Work out the finished part from the listing and answer in its coordinate system (mm). Face numbers are marked on the shaded views. Round coordinates to 2 decimals unless told otherwise and drop trailing zeros. Loops run counter-clockwise (first coordinate to the right, second up) from the corner with the lowest first, then second, coordinate; pieces in that order, holes last. Notation, with made-up numbers: M 69,19.5 L 75,19.5 A14 cw 75,35.5 Z; hole C -14,-11.5 d8. An arc over 180 degrees is marked long. One line per item, written item: value.
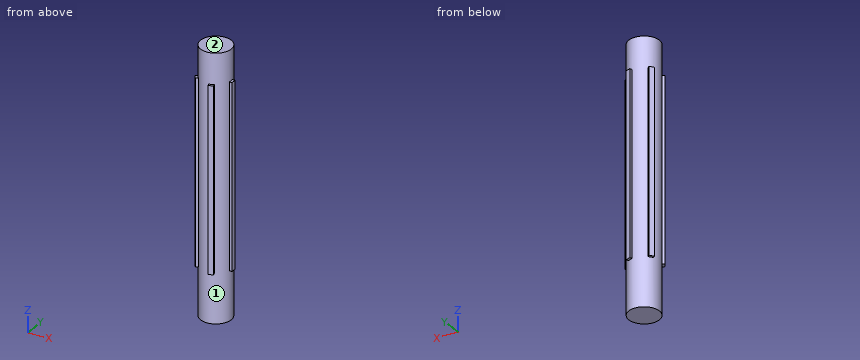
```python
from build123d import *

# Parameters (mm, degrees)
SKETCH1_R           = 12.5
BOSS_EXTRUDE1_DEPTH = 215
BOSS_EXTRUDE2_START = 40
BOSS_EXTRUDE2_DEPTH = 150
CIRPATTERN1_COUNT   = 5


with BuildPart() as part:
    # Sketch1 → Boss-Extrude1 (new body)
    with BuildSketch(Plane.XY):
        Circle(SKETCH1_R)
    extrude(amount=BOSS_EXTRUDE1_DEPTH)

    # Sketch1_3 → Boss-Extrude2 (add)
    with BuildSketch(Plane.XY.offset(BOSS_EXTRUDE2_START)):
        with BuildLine():
            Line((14.5, -2), (14.5, 2))
            Line((14.5, 2), (12.338962679, 2))
            ThreePointArc((12.338962679, 2), (12.459675628, 1.00323639), (12.5, 0))
            ThreePointArc((12.5, 0), (12.459675628, -1.00323639), (12.338962679, -2))
            Line((12.338962679, -2), (14.5, -2))
        make_face()
    boss_extrude2 = extrude(amount=BOSS_EXTRUDE2_DEPTH)

    # CirPattern1: Boss-Extrude2 ×5 about axis
    cirpattern1_axis = Axis((0, 0, 0), (0, 0, 1))
    for i in range(1, CIRPATTERN1_COUNT):
        add(boss_extrude2.rotate(cirpattern1_axis, i * 360 / CIRPATTERN1_COUNT))


solid = part.part
```
1) Find section C-C (x = 0). Give the vertices of the cut face in (y, z).
Check values:
outline: M -12.5,0 L 12.5,0 L 12.5,215 L -12.5,215 Z
2) Find section B-B (z = 110). Give the vertices of the cut face in (x, y).
Check values:
outline: M -12.91,-6.9 L -10.56,-10.14 L -8.81,-8.87 A12.5 ccw 1.91,-12.35 L 2.58,-14.41 L 6.38,-13.17 L 5.72,-11.12 A12.5 ccw 12.34,-2 L 14.5,-2 L 14.5,2 L 12.34,2 A12.5 ccw 5.72,11.12 L 6.38,13.17 L 2.58,14.41 L 1.91,12.35 A12.5 ccw -8.81,8.87 L -10.56,10.14 L -12.91,6.9 L -11.16,5.63 A12.5 ccw -11.16,-5.63 Z
3) Each of these flat-tipped pins is pushed along its axis until it touches: pin 1 (3.5 mm diameter, centred on x = 3.5, y = 13, fed in from -Z); pin 2 (12 mm diameter, centred on x = 11.5, z = 53, fed in from -Y); pin 3 (0.6 mm diameter, centred on x = 13.5, z = 127, fed in from +Y); pin 4 (1 mm diameter, centred on y = -6.5, z = 148.5, fed in from +X). Where does it stop, or does it pass through?
Check values:
pin 1: z = 0
pin 2: y = -13.46
pin 3: y = 2
pin 4: x = 10.97
4) Find the intervals of material crossed by probe 1 along X at (y, z) = (0.5, 74); probe 2 along Y at (x, z) = (-11.5, 186.5); probe 3 along Y at (x, z) = (-2, 184), in increasing order. Write a range as from..to.
Check values:
probe 1: -12.49..14.5
probe 2: -8.84..-5.88, -4.9..4.9, 5.88..8.84
probe 3: -12.34..12.34
5) Find section A-A (y = 0). Give the vertices of the cut face in (x, z), then the cut area to 4 significant figures.
Check values:
outline: M -12.5,0 L 12.5,0 L 12.5,40 L 14.5,40 L 14.5,190 L 12.5,190 L 12.5,215 L -12.5,215 Z
area: 5,675 mm2
6) The mould has two halves that part along Y. Classify the marked faces 1 and 2: +Y half, -Y half, draft (parallel to the pull), parting line (faces both ways), or undercut.
Check values:
face 1: undercut
face 2: draft
7) Find section D-D (z = 17). Give the vertices of the cut face in (x, y), then the cut area to 3 significant figures.
Check values:
outline: C 0,0 d25
area: 491 mm2
